CAD build for the part. Positions are in the model's coordinates, mm. Face numbers are marked on the shaded views. A direction names the side the tool comes from. Coordinates: 2 decimals unless noted, no trailing zeros. Order: outer loops, then holes, each group sorted by start corner. A loop starts at its lowest first (then second) coordinate and runs counter-clockwise, first axis right, second up. Notation, with made-up numbers: (49.5, 51.25) -> (73.5, 51.25) arc R21 ccw to (73.5, 76.25) -> close; hole circle Ø1 at (75, -21.5). An arc over 180 degrees is marked (long way). Use one line per item in the form item = value. Start each with the question number.
from build123d import *

# Parameters (mm, degrees)
PROFILE_SKETCH_R             = 12.7
PROFILE_EXTRUDE_DEPTH        = 6.35
GAP_SKETCH_W                 = 1.27
GAP_SKETCH_H                 = 17.15262
GAP_CUT_DEPTH                = 7.35
CROSSBOLT_HOLE_SKETCH_R      = 1.5875
CROSSBOLT_HOLE_CUT_DEPTH     = 10
NUT_CAPTURE_POCKET_SKETCH_W  = 4.8
NUT_CAPTURE_POCKET_SKETCH_H  = 5.627
NUT_CAPTURE_POCKET_CUT_DEPTH = 6.35
MOUNTING_HOLE_SKETCH_R       = 1.5875
MOUNTING_HOLE_CUT_DEPTH      = 6.2
LIGHTENING_POCKET_CUT_DEPTH  = 6.35


with BuildPart() as part:
    # Profile Sketch → Profile Extrude (new body)
    with BuildSketch(Plane.XY):
        with BuildLine():
            Line((-15.875, 0), (-15.875, 15.875))
            Line((-15.875, 15.875), (-23.124999989, 15.875))
            Line((-23.124999989, 15.875), (-23.124999989, 22.075))
            Line((-23.124999989, 22.075), (23.124999989, 22.075))
            Line((23.124999989, 22.075), (23.124999989, 15.875))
            Line((23.124999989, 15.875), (15.875, 15.875))
            Line((15.875, 15.875), (15.875, 0))
            ThreePointArc((15.875, 0), (12.872269128, -9.290872537), (5, -15.067037698))
            Line((5, -15.067037698), (5, -24.592037698))
            Line((5, -24.592037698), (-5, -24.592037698))
            Line((-5, -24.592037698), (-5, -15.067037698))
            ThreePointArc((-5, -15.067037698), (-12.872269128, -9.290872537), (-15.875, 0))
        make_face()
        Circle(PROFILE_SKETCH_R, mode=Mode.SUBTRACT)
    extrude(amount=PROFILE_EXTRUDE_DEPTH)

    # Gap Sketch → Gap Cut (cut, through all)
    with BuildSketch(Plane.XY.offset(6.35)):
        with Locations((0, -17.526)):
            Rectangle(GAP_SKETCH_W, GAP_SKETCH_H)
    extrude(amount=-GAP_CUT_DEPTH, mode=Mode.SUBTRACT)

    # Crossbolt Hole Sketch → Crossbolt Hole Cut (cut)
    with BuildSketch(Plane(origin=(5, 0, 0), x_dir=(0, 0, -1), z_dir=(1, 0, 0))):
        with Locations((-3.175, -19.829537698)):
            Circle(CROSSBOLT_HOLE_SKETCH_R)
    extrude(amount=-CROSSBOLT_HOLE_CUT_DEPTH, mode=Mode.SUBTRACT)

    # Nut Capture Pocket Sketch → Nut Capture Pocket Cut (cut)
    with BuildSketch(Plane.XY.offset(6.35)):
        with Locations((-5, -19.829537698)):
            Rectangle(NUT_CAPTURE_POCKET_SKETCH_W, NUT_CAPTURE_POCKET_SKETCH_H)
    extrude(amount=-NUT_CAPTURE_POCKET_CUT_DEPTH, mode=Mode.SUBTRACT)

    # Mounting Hole Sketch → Mounting Hole Cut (cut)
    with BuildSketch(Plane.XZ.offset(-15.875)):
        with Locations((19.499999994, 3.175)):
            Circle(MOUNTING_HOLE_SKETCH_R)
        with Locations((-19.499999995, 3.175)):
            Circle(MOUNTING_HOLE_SKETCH_R)
    extrude(amount=-MOUNTING_HOLE_CUT_DEPTH, mode=Mode.SUBTRACT)

    # Lightening Pocket Sketch → Lightening Pocket Cut (cut)
    with BuildSketch(Plane.XY.offset(6.35)):
        with BuildLine():
            Line((12.7, 18.9), (-12.7, 18.9))
            Line((-12.7, 18.9), (-12.7, 9.525))
            ThreePointArc((-12.7, 9.525), (0, 15.875), (12.7, 9.525))
            Line((12.7, 9.525), (12.7, 18.9))
        make_face()
    extrude(amount=-LIGHTENING_POCKET_CUT_DEPTH, mode=Mode.SUBTRACT)


solid = part.part
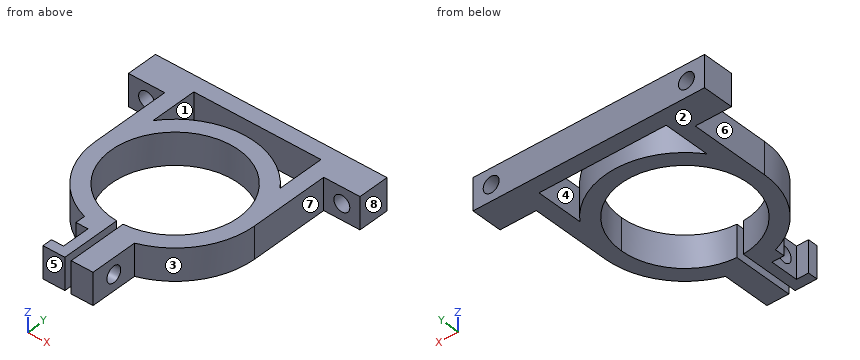
1) Cut at D-D on z = 2.5. Count the separate pieces of the cut face and the enclosed holes in it, then the cut area to 3 significant figures.
2) Two-plate mould, pull along Y, no slides. Class the marked faces 1, 2 and 3: released by +Y, released by -Y, zero draft, split by the parting line, or undercut.
3) Cut at A-A on x = 0. Give the cut face in (y, z) (3 decimals), then the cut area to 3 significant figures.
4) Cut at B-B on y = 1. Give the cut face in (x, z) (3 decimals), then the cut area to 3 significant figures.
5) Cut at C-C on y = 11. Give the cut face in (x, z) (3 decimals).
6) Drop flat-ended pins along their axis: P1, Ø1.6, axis at y = -15.5, z = 4.5, coming from the -X side; P2, Ø1.7, axis at y = -19.5, z = 3.5, coming from the -X side; P3, Ø1.9, axis at y = 15.5, z = 2, coming from the -X side (3 decimals); P4, Ø1, axis at x = 13, z = 4.5, coming from the -Y side. Give the stop position or say it passes through.
7) 3-axis set-ups, long thin cutter, end or side, ignore diameter. For the marked faces 4, 5, 6, 7 and 8: which of +Z, -Z, +X, -X, +Y, -Y reach the whole face in a straight line?
8) Probe L1, parallel to X at y = -16, z = 2.5 (3 decimals); L2, parallel to Y at x = 1, z = 4.5 (3 decimals); L3, parallel to Y at x = 0.5, z = 1 (3 decimals). List the from-to ranges inside material, lowest first.
Values follow:
q1.separate_pieces = 5
q1.enclosed_holes = 1
q1.area = 562 mm^2
q2.face_1 = undercut
q2.face_2 = zero draft
q2.face_3 = released by -Y
q3.outline = (12.7, 0) -> (15.875, 0) -> (15.875, 6.35) -> (12.7, 6.35) -> close; (18.9, 0) -> (22.075, 0) -> (22.075, 6.35) -> (18.9, 6.35) -> close
q3.area = 40.3 mm^2
q4.outline = (-15.875, 0) -> (-12.661, 0) -> (-12.661, 6.35) -> (-15.875, 6.35) -> close; (12.661, 0) -> (15.875, 0) -> (15.875, 6.35) -> (12.661, 6.35) -> close
q4.area = 40.8 mm^2
q5.outline = (-15.875, 0) -> (-12.7, 0) -> (-12.7, 6.35) -> (-15.875, 6.35) -> close; (-11.446, 0) -> (-6.347, 0) -> (-6.347, 6.35) -> (-11.446, 6.35) -> close; (6.347, 0) -> (11.446, 0) -> (11.446, 6.35) -> (6.347, 6.35) -> close; (12.7, 0) -> (15.875, 0) -> (15.875, 6.35) -> (12.7, 6.35) -> close
q6.P1 = -5.99
q6.P2 = through
q6.P3 = -23.125
q6.P4 = -9.79
q7.face_4 = +Z, -Z
q7.face_5 = +Z, -Z, +X, -X, -Y
q7.face_6 = +Z, -Z, -X, -Y
q7.face_7 = +Z, -Z, +X, -Y
q7.face_8 = +Z, -Z, +X, +Y, -Y
q8.L1 = -5 to -0.635, 0.635 to 5
q8.L2 = -24.592 to -20.704, -18.955 to -12.661, 12.661 to 15.843, 18.9 to 22.075
q8.L3 = 12.69 to 15.867, 18.9 to 22.075
